The listing builds one solid part. Answer for the finished solid, in the listing's coordinates (mm). Face numbers are marked on the shaded views. A direction names the side the tool comes from. Give positions to 0.01 mm unless a question says otherwise; leave off trailing zeros. Write each loop counter-clockwise with the first axis right and the second up, starting at its lowest first coordinate (ties: lowest second). Pieces come first, ordered by that corner, then holes. Notation, with made-up numbers: (43, -0.5) -> (88, -0.5) arc R20 cw to (88, 19.5) -> close; hole circle Ø5 at (52, 86.5). An arc over 180 degrees is marked (long way). Put each result on its own line as item: value. Start each with the question number.
1) A cutting plane is placed at B-B (y = -6.35). Write down the section's boundary in (x, z) (3 decimals), then the cut area to 3 significant figures.
2) For a pull along X with two mould halves and no side action, classify the marked faces 1, 2 and 3 as released by +X, released by -X, zero draft, split by the parting line, or undercut.
3) A cutting plane is placed at A-A (z = -6.35). Write down the section's boundary in (x, y) (3 decimals).
4) Find the intervals of material crossed by line 1 along Y through (x, z) = (25.4, -6.25) (3 decimals); line 2 along Z through (x, y) = (16, -23.5); line 3 along Z through (x, y) = (31, -9.75), in increasing order. Write a range as from..to.
5) For the marked faces 4, 5 and 6, determine the directions among +Z, -Z, +X, -X, +Y, -Y from which every point of the face is accessible in a straight line to the end or side of a thin tool.
6) A cutting plane is placed at D-D (y = -15.5). Write down the section's boundary in (x, z) (3 decimals), then the cut area to 3 significant figures.
7) A cutting plane is placed at C-C (x = 25.4). Write down the section's boundary in (y, z) (3 decimals).
8) Flat-ended cylindrical pins translate along their axes: pin 1 Ø9.5 at (y, z) = (-7.5, -9) entering from +X; pin 2 Ø1 at (x, y) = (17, -11) entering from -Z; pin 3 Ø10 at (x, z) = (9.652, -6.35) entering from -Y. Find the tip coordinate at first contact, or state that the pin passes through.
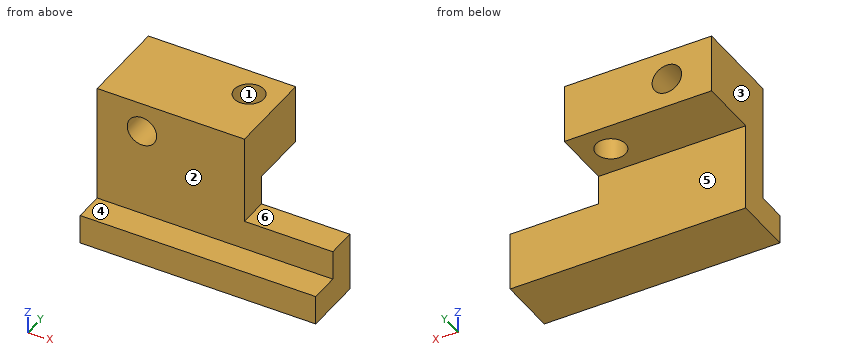
from build123d import *

# Parameters (mm, degrees)
F0_W     = 19.05
F0_H     = 12.7
F1_DEPTH = 31.75
F2_W     = 6.35
F2_H     = 6.35
F3_DEPTH = 31.75
F5_DEPTH = 50.8
F6_R     = 3.175
F7_DEPTH = 31.751
F8_R     = 3.175
F9_DEPTH = 19.051


with BuildPart() as f1:
    # F0 (on Right) → F1 (new body)
    with BuildSketch(Plane.YZ):
        with Locations((-9.525, -6.35)):
            Rectangle(F0_W, F0_H)
    extrude(amount=F1_DEPTH)

    # F2 (on face) → F3 (join)
    with BuildSketch(Plane(origin=(0, 0, 0), x_dir=(0, -1, 0), z_dir=(-1, 0, 0))):
        with Locations((15.875, -15.875)):
            Rectangle(F2_W, F2_H)
    extrude(amount=-F3_DEPTH)

    # F4 (on face) → F5 (join)
    with BuildSketch(Plane(origin=(0, 0, 0), x_dir=(0, -1, 0), z_dir=(-1, 0, 0))):
        Polygon((19.05, -25.4), (19.05, -19.05), (12.7, -19.05), (12.7, -31.75), (25.4, -31.75), (25.4, -25.4), align=None)
    extrude(amount=-F5_DEPTH)

    # F6 (on face) → F7 (cut, through all)
    with BuildSketch(Plane.XY):
        with Locations((25.4, -6.35)):
            Circle(F6_R)
    extrude(amount=-F7_DEPTH, mode=Mode.SUBTRACT)

    # F8 (on face) → F9 (cut, through all)
    with BuildSketch(Plane.XZ.offset(19.05)):
        with Locations((9.652, -6.35)):
            Circle(F8_R)
    extrude(amount=-F9_DEPTH, mode=Mode.SUBTRACT)


solid = f1.part
Reply:
1. outline: (0, -12.7) -> (22.225, -12.7) -> (22.225, 0) -> (0, 0) -> close; (28.575, -12.7) -> (31.75, -12.7) -> (31.75, 0) -> (28.575, 0) -> close; hole circle Ø6.35 at (9.652, -6.35)
1. area: 291 mm2
2. face 1: undercut
2. face 2: zero draft
2. face 3: released by -X
3. outline: (0, -19.05) -> (6.477, -19.05) -> (6.477, 0) -> (0, 0) -> close; (12.827, -19.05) -> (31.75, -19.05) -> (31.75, 0) -> (12.827, 0) -> close; hole circle Ø6.35 at (25.4, -6.35)
4. line 1: y = -19.05..-9.525, -3.175..0
4. line 2: z = -31.75..-25.4
4. line 3: z = -12.7..0
5. face 4: +Z, +X, -X, -Y
5. face 5: -Z, +X, -X, +Y
5. face 6: +Z, +X, +Y, -Y
6. outline: (0, -31.75) -> (50.8, -31.75) -> (50.8, -19.05) -> (31.75, -19.05) -> (31.75, 0) -> (0, 0) -> close; hole circle Ø6.35 at (9.652, -6.35)
6. area: 1,220 mm2
7. outline: (-25.4, -31.75) -> (-12.7, -31.75) -> (-12.7, -12.7) -> (-9.525, -12.7) -> (-9.525, 0) -> (-19.05, 0) -> (-19.05, -25.4) -> (-25.4, -25.4) -> close; (-3.175, -12.7) -> (0, -12.7) -> (0, 0) -> (-3.175, 0) -> close
8. pin 1: stops at x = 31.75
8. pin 2: stops at z = -12.7
8. pin 3: stops at y = -19.05
